Build history of the part. All positions in model axes, mm. A direction names the side the tool comes from. Round coordinates to 2 decimals unless told otherwise and drop trailing zeros. Order: outer loops, then holes, each group sorted by start corner. A loop starts at its lowest first (then second) coordinate and runs counter-clockwise, first axis right, second up. Notation, with made-up numbers: (20, 32) -> (54, 32) arc R24 cw to (54, 51) -> close; hole circle Ø8 at (31.25, 46). An arc over 180 degrees is marked (long way). Answer as a JSON object with one key per item and string values.
from build123d import *

# Parameters (mm, degrees)
SKETCH1_W           = 9
SKETCH1_H           = 2
BOSS_EXTRUDE1_DEPTH = 15
CUT_EXTRUDE1_START  = -31
SKETCH2_W           = 8
SKETCH2_H           = 0.5
CUT_EXTRUDE1_DEPTH  = 32


with BuildPart() as part:
    # Sketch1 → Boss-Extrude1 (new body, symmetric)
    with BuildSketch(Plane(origin=(0, 0, 0), x_dir=(1, 0, 0), z_dir=(0, 1, 0))):
        Rectangle(SKETCH1_W, SKETCH1_H)
    extrude(amount=BOSS_EXTRUDE1_DEPTH, both=True)

    # Sketch2 → Cut-Extrude1 (cut)
    with BuildSketch(Plane(origin=(0, 15, 0), x_dir=(1, 0, 0), z_dir=(0, 1, 0)).offset(CUT_EXTRUDE1_START)):
        with Locations((0, 0.5)):
            Rectangle(SKETCH2_W, SKETCH2_H)
    cut_extrude1 = extrude(amount=CUT_EXTRUDE1_DEPTH, mode=Mode.SUBTRACT)

    # Mirror1: Cut-Extrude1 across plane
    add(cut_extrude1.mirror(Plane.XY), mode=Mode.SUBTRACT)


solid = part.part
1) Which spindle directions (+Z, -Z, +X, -X, +Y, -Y) get a long thin tool onto all of the face, cutting with end or side? Do faces 4 (the face through (0, 0, 0.75)), 5 (the face through (0, 15, 0)). Say none if no direction does.
Checked values:
{"face 4": "+Y, -Y", "face 5": "+Z, -Z, +X, -X, +Y"}
2) Pull direction Z, two halves, no side cores. Call faces 1 (the face through (0, 0, -0.75)), 2 (the face through (-4.5, 0, 0)), 3 (the face through (0, 0, 1)): pulls with the +Z half, pulls with the -Z half, needs draft (parallel to the pull), parting line crosses it, or undercut.
Checked values:
{"face 1": "undercut", "face 2": "needs draft", "face 3": "pulls with the +Z half"}
3) Cut at A-A, the plane x = 3. Give the cut face in (y, z).
Checked values:
{"outline": "(-15, -1) -> (15, -1) -> (15, -0.75) -> (-15, -0.75) -> close; (-15, -0.25) -> (15, -0.25) -> (15, 0.25) -> (-15, 0.25) -> close; (-15, 0.75) -> (15, 0.75) -> (15, 1) -> (-15, 1) -> close"}
4) Probe L1, parallel to Z at x = 2.25, y = 7; L2, parallel to X at y = 9.75, z = -0.5. List the from-to ranges inside material, lowest first. Write a range as from..to.
Checked values:
{"L1": "z = -1..-0.75, -0.25..0.25, 0.75..1", "L2": "x = -4.5..-4, 4..4.5"}
5) Cut at B-B, the plane y = -9. Give the cut face in (x, z).
Checked values:
{"outline": "(-4.5, -1) -> (4.5, -1) -> (4.5, 1) -> (-4.5, 1) -> close; hole (-4, -0.75) -> (4, -0.75) -> (4, -0.25) -> (-4, -0.25) -> close; hole (-4, 0.25) -> (4, 0.25) -> (4, 0.75) -> (-4, 0.75) -> close"}
